Autodesk Inventor part; units mm, degrees
ref_plane "YZ Plane" through (0, 0, 0) normal (1, 0, 0) x (0, 1, 0)
ref_plane "XZ Plane" through (0, 0, 0) normal (0, 1, 0) x (-1, 0, 0)
ref_plane "XY Plane" through (0, 0, 0) normal (0, 0, 1) x (1, 0, 0)
sketch "Sketch1" plane through (0, 0, 0) normal (0, 0, 1) x (1, 0, 0)
  circle A0 centre (0, 0) radius 45.212
  dimension "d0" = 90.424
extrude "Extrusion1" add sketch "Sketch1" along normal blind 4.7625
sketch "Sketch2" plane through (0, 0, 0) normal (0, 0, -1) x (-1, 0, 0)
  circle A0 centre (0, 0) radius 25.4
  dimension "d3" = 50.8
extrude "Extrusion2" cut sketch "Sketch2" against normal blind 4.7625
sketch "Sketch4" plane through (0, 0, 4.7625) normal (0, 0, 1) x (1, 0, 0)
  circle A0 centre (0, 41.91) radius 1.905
  circle A1 centre (-36.2951, 20.955) radius 1.905
  circle A2 centre (-36.2951, -20.955) radius 1.905
  circle A3 centre (0, -41.91) radius 1.905
  circle A4 centre (36.2951, -20.955) radius 1.905
  circle A5 centre (36.2951, 20.955) radius 1.905
  point P0 (0, 0)
  dimension "d14" = 3.81
  dimension "d15" = 41.91
  dimension "d18" = 360
extrude "Extrusion4" cut sketch "Sketch4" against normal blind 25.4
sketch "Sketch5" plane through (0, 0, 4.7625) normal (0, 0, 1) x (1, 0, 0)
  circle A0 centre (20.795, 25.8191) radius 3.175
  line L0 (0, 0) -> (0, 18.2107)
  circle A1 centre (-20.795, 25.8191) radius 3.175
  dimension "d22" = 6.35
  dimension "d23" = 25.8191
  dimension "d24" = 20.795
extrude "Extrusion5" cut sketch "Sketch5" against normal blind 25.4
sketch "Sketch6" plane through (0, 0, 4.7625) normal (0, 0, 1) x (1, 0, 0)
  circle A0 centre (20.795, 25.8191) radius 3.175
  circle A1 centre (-20.795, 25.8191) radius 3.175
  circle A2 centre (36.2951, -20.955) radius 1.905
  circle A3 centre (-36.2951, -20.955) radius 1.905
  circle A4 centre (0, 41.91) radius 1.905
  circle A5 centre (-36.2951, 20.955) radius 1.905
  circle A6 centre (0, -41.91) radius 1.905
  circle A7 centre (36.2951, 20.955) radius 1.905
  circle A8 centre (0, 0) radius 25.4
  circle A9 centre (0, 0) radius 45.212
  circle A10 centre (0, 0) radius 36.327
  circle A11 centre (-20.795, 25.8191) radius 3.175
extrude "Extrusion6" cut sketch "Sketch6" against normal blind 25.4 contours A10
properties part number "AluminumSealingDisc" material "Aluminum 6061"
Build history of the part. All positions in model axes, mm. Give positions to 0.01 mm unless a question says otherwise; leave off trailing zeros. Loops run counter-clockwise (first coordinate to the right, second up) from the corner with the lowest first, then second, coordinate; pieces in that order, holes last. Notation, with made-up numbers: (-8, 0) -> (27, 0) arc R17 cw to (27, 14) -> close; hole circle Ø4 at (46, -39). An arc over 180 degrees is marked (long way). Answer in a Markdown table with one row per item.
Item 1: Mould opens along Y. For faces 1 (the flat face through (-34, 14, 0)), 2 (the cylindrical face through (-0.41, -43.77, 2.41)), 3 (the cylindrical face through (43.124, -13.58, 2.348)) say: pulls with the +Y half, pulls with the -Y half, needs draft (parallel to the pull), parting line crosses it, or undercut.
Findings below:
| item | result |
|---|---|
| face 1 | needs draft |
| face 2 | undercut |
| face 3 | parting line crosses it |
Item 2: Slice it at C-C on x = -25.5. Write the cut outline in (y, z).
Findings below:
| item | result |
|---|---|
| outline | (-37.33, 0) -> (-25.87, 0) -> (-25.87, 4.76) -> (-37.33, 4.76) -> close; (25.87, 0) -> (37.33, 0) -> (37.33, 4.76) -> (25.87, 4.76) -> close |
Item 3: Slice it at D-D on z = 2.6. Write the cut outline in (x, y) (3 decimals).
Findings below:
| item | result |
|---|---|
| outline | circle Ø90.424 at (0, 0); hole circle Ø3.81 at (-36.295, -20.955); hole circle Ø3.81 at (-36.295, 20.955); hole circle Ø72.654 at (0, 0); hole circle Ø3.81 at (0, -41.91); hole circle Ø3.81 at (0, 41.91); hole circle Ø3.81 at (36.295, -20.955); hole circle Ø3.81 at (36.295, 20.955) |
Item 4: Flat gauge pins, fed straight in: P1, Ø6, axis at x = -36.3, y = -20.96, coming from the -Z side; P2, Ø1.5, axis at y = 11, z = 3.5, coming from the -X side; P3, Ø2, axis at y = -22, z = 2.5, coming from the -X side; P4, Ø1.5, axis at x = 27.5, z = 4.5, coming from the -Y side. Where does each tip first touch, or does it go through?
Findings below:
| item | result |
|---|---|
| P1 | stops at z = 0 |
| P2 | stops at x = -44.03 |
| P3 | stops at x = -40.04 |
| P4 | stops at y = -36.45 |
Item 5: Slice it at B-B on y = 0. Write the cut outline in (x, z), plus the area to 3 significant figures.
Findings below:
| item | result |
|---|---|
| outline | (-45.21, 0) -> (-36.33, 0) -> (-36.33, 4.76) -> (-45.21, 4.76) -> close; (36.33, 0) -> (45.21, 0) -> (45.21, 4.76) -> (36.33, 4.76) -> close |
| area | 84.6 mm² |
Item 6: Slice it at A-A on x = 0. Write the cut outline in (y, z) (1 decimal), plus the area to 3 significant figures.
Findings below:
| item | result |
|---|---|
| outline | (-45.2, 0) -> (-43.8, 0) -> (-43.8, 4.8) -> (-45.2, 4.8) -> close; (-40, 0) -> (-36.3, 0) -> (-36.3, 4.8) -> (-40, 4.8) -> close; (36.3, 0) -> (40, 0) -> (40, 4.8) -> (36.3, 4.8) -> close; (43.8, 0) -> (45.2, 0) -> (45.2, 4.8) -> (43.8, 4.8) -> close |
| area | 48.3 mm² |
Item 7: Probe line 1 along Y through (x, z) = (0, 1.6) (3 decimals); line 2 along Y through (x, z) = (-37, 3.55); line 3 along Y through (x, z) = (-1.5, 4.1). List the from-to ranges inside material, lowest first. Write a range as [from, to].
Findings below:
| item | result |
|---|---|
| line 1 | y = [-45.212, -43.815], [-40.005, -36.327], [36.327, 40.005], [43.815, 45.212] |
| line 2 | y = [-25.98, -22.72], [-19.19, 19.19], [22.72, 25.98] |
| line 3 | y = [-45.19, -43.08], [-40.74, -36.3], [36.3, 40.74], [43.08, 45.19] |
